The listing builds one solid part. Answer for the finished solid, in the listing's coordinates (mm). Face numbers are marked on the shaded views. A direction names the side the tool comes from. Give positions to 0.01 mm unless a question says otherwise; leave off trailing zeros. Loops run counter-clockwise (first coordinate to the right, second up) from the corner with the lowest first, then second, coordinate; pieces in that order, holes last. Notation, with made-up numbers: M 31.5,-9 L 46.5,-9 A7 ccw 46.5,-2 Z; hole C 80,26.25 d3. An arc over 180 degrees is marked long. One line per item, written item: value. Start each with the question number.
Q1. A cutting plane is placed at C-C, the plane y = 9. Determine the outline of the cut face in (x, z) (3 decimals), and give its area (3 significant figures).
Q2. A cutting plane is placed at D-D, the plane x = -21.5. Determine the outline of the cut face in (y, z).
Q3. The mould has two halves that part along Y. Classify the marked faces 1, 2 and 3: +Y half, -Y half, draft (parallel to the pull), parting line (faces both ways), or undercut.
Q4. Flat-ended cylindrical pins translate along their axes: pin 1 (2 mm diameter, centred on x = -3.5, y = 6.5, fed in from -Z); pin 2 (2 mm diameter, centred on x = 0, y = 6, fed in from +Z); pin 3 (4 mm diameter, centred on y = 8.5, z = -11, fed in from +X). Find the tip coordinate at first contact, or state that the pin passes through.
Q5. Consider L1, parallel to Y at x = -12, z = -20; L2, parallel to Z at x = -19, y = 9.5; L3, parallel to Z at x = 16.5, y = 6.75. Determine where each line is inside the solid, lowest interval first.
Q6. For the marked faces 4 and 5, determine the directions among +Z, -Z, +X, -X, +Y, -Y from which every point of the face is accessible in a straight line to the end or side of a thin tool.
Autodesk Fusion 360 part; units mm, degrees
sketch "Base" plane through (0, 0, 0) normal (0, 1, 0) x (1, 0, 0)
  circle A0 centre (0, 0) radius 25.4
  dimension "d1" = 50.8
extrude "Extrude1" add sketch "Base" along normal blind 12.7 makes body 1
sketch "Relief" plane through (0, 12.7, 0) normal (0, 1, 0) x (-1, 0, 0)
  circle A0 centre (0, 0) radius 25.4
  circle A1 centre (0, -25.4) radius 9.525
  dimension "d4" = 19.05
extrude "Extrude2" cut sketch "Relief" against normal blind 6.35 contours A0 A1 | A0 A1 picked at (1.7493, -22.2335) picked at (2.3346, -28.2419) bodies 1
sketch "Boss Ref" plane through (0, 12.7, 0) normal (0, 1, 0) x (-1, 0, 0)
  arc A0 (9.3561, -23.6141) -> (-9.3561, -23.6141) centre (0, -25.4) ccw
  arc A1 (9.3561, -23.6141) -> (-9.3561, -23.6141) centre (0, 0) ccw
  circle A2 centre (0, -10.795) radius 4.7625
  circle A3 centre (0, -10.795) radius 2.5527
  dimension "d7" = 9.525
  dimension "d8" = 10.795
  dimension "d9" = 5.1054
sketch "Revolve Cut1" plane through (0, 0, 0) normal (1, 0, 0) x (0, 0, -1)
  line L0 (25.4, 0) -> (25.4, 6.35)
  line L1 (-25.4, 12.7) -> (-25.4, 0)
  line L2 (15.875, 6.35) -> (23.6141, 6.35)
  line L3 (25.4, 6.35) -> (22.225, 6.35)
  line L4 (22.225, 7.9375) -> (25.4, 7.9375)
  line L5 (25.4, 7.9375) -> (25.4, 6.35)
  line L6 (22.225, 7.9375) -> (22.225, 6.35)
  dimension "d12" = 3.175
  dimension "d13" = 1.5875
revolve "Revolve1" cut sketch "Revolve Cut1" angle 360 about axis through (0, 1.75, 0) along (0, 1, 0) bodies 1
sketch "Sketch5" plane through (0, 12.7, 0) normal (0, 1, 0) x (-1, 0, 0)
  arc A0 (9.3561, -23.6141) -> (-9.3561, -23.6141) centre (0, -25.4) ccw
  arc A1 (9.3561, -23.6141) -> (-9.3561, -23.6141) centre (0, 0) ccw
  arc A2 (-8.2489, -20.6375) -> (-9.3561, -23.6141) centre (0, -25.4) ccw
  arc A3 (9.3561, -23.6141) -> (-9.3561, -23.6141) centre (0, 0) ccw
  arc A4 (9.3561, -23.6141) -> (8.2489, -20.6375) centre (0, -25.4) ccw
  arc A5 (8.2489, -20.6375) -> (-8.2489, -20.6375) centre (0, 0) ccw
  line L0 (0, -15.875) -> (-6.35, -9.525)
  line L1 (0, -15.875) -> (6.35, -9.525)
  line L2 (6.35, -9.525) -> (-6.35, -9.525)
  line L3 (0, -9.525) -> (0, -15.875) construction
  line L4 (6.35, -3.175) -> (-6.35, -3.175)
  line L5 (6.35, -9.525) -> (6.35, -3.175)
  line L6 (-6.35, -9.525) -> (-6.35, -3.175)
  line L7 (-6.35, -3.175) -> (-12.7, -3.175)
  line L8 (-12.7, -3.175) -> (-6.35, -9.525)
  line L9 (6.35, -9.525) -> (12.7, -3.175)
  line L10 (12.7, -3.175) -> (6.35, -3.175)
  dimension "d15" = 6.35
  dimension "d16" = 45
  dimension "d17" = 6.35
ref_plane "WorkPlane1" through (0, 0, -23.6141) normal (0, 0, 1) x (1, 0, 0)
sketch "Loft Profile 2" plane through (0, 12.7, 0) normal (0, 1, 0) x (-1, 0, 0)
  arc A0 (9.3561, -23.6141) -> (-9.3561, -23.6141) centre (0, -25.4) ccw
  arc A1 (9.3561, -23.6141) -> (-9.3561, -23.6141) centre (0, 0) ccw
  line L0 (4.7625, 8.255) -> (-4.7625, 8.255)
  arc A2 (-4.7625, 8.255) -> (-4.7625, -8.255) centre (-4.7625, 0) ccw
  line L1 (-4.7625, -8.255) -> (4.7625, -8.255)
  arc A3 (4.7625, -8.255) -> (4.7625, 8.255) centre (4.7625, 0) ccw
  line L2 (4.7625, 0) -> (-4.7625, 0) construction
  dimension "d19" = 9.525
  dimension "d20" = 8.255
sketch "Loft Profile 1" plane through (0, 0, 0) normal (0, -1, 0) x (1, 0, 0)
  circle A0 centre (0, 0) radius 25.4
  circle A1 centre (0, 0) radius 6.35
  dimension "d21" = 12.7
sketch "Sweep Profile" plane through (0, 0, 0) normal (0, -1, 0) x (1, 0, 0)
  circle A0 centre (0, 0) radius 25.4
  circle A1 centre (0, 0) radius 19.05
  dimension "d22" = 38.1
sketch "Sweep Path" plane through (0, 0, 0) normal (0, 0, 1) x (1, 0, 0)
  line L0 (0, 0) -> (0, -63.5)
  arc A0 (0, -63.5) -> (50.1381, -135.1046) centre (76.2, -63.5) ccw
  line L1 (50.1381, -135.1046) -> (169.479, -178.5411)
  dimension "d23" = 76.2
  dimension "d24" = 63.5
  dimension "d25" = 127
  dimension "d26" = 110
sketch "Hole Loc1" plane through (0, 12.7, 0) normal (0, 1, 0) x (-1, 0, 0)
  arc A0 (9.3561, -23.6141) -> (-9.3561, -23.6141) centre (0, -25.4) ccw
  arc A1 (9.3561, -23.6141) -> (-9.3561, -23.6141) centre (0, 0) ccw
  line L0 (0, 0) -> (0, -15.875) construction
  line L1 (0, 0) -> (-11.2253, -11.2253) construction
  point P0 (-11.2253, -11.2253)
  point P1 (11.2253, -11.2253)
  point P2 (11.2253, 11.2253)
  point P3 (-11.2253, 11.2253)
  dimension "d27" = 45
  dimension "d29" = 360
sketch "Extrude" plane through (0, 12.7, 0) normal (0, 1, 0) x (-1, 0, 0)
  arc A0 (9.3561, -23.6141) -> (-9.3561, -23.6141) centre (0, -25.4) ccw
  arc A1 (9.3561, -23.6141) -> (-9.3561, -23.6141) centre (0, 0) ccw
  line L0 (3.175, -16.4197) -> (-3.175, -16.4197)
  line L1 (-3.175, -16.4197) -> (-3.175, -9.525)
  line L2 (-3.175, -9.525) -> (3.175, -9.525)
  line L3 (3.175, -9.525) -> (3.175, -16.4197)
  line L4 (0, -9.525) -> (0, -15.875) construction
  dimension "d30" = 6.35
  dimension "d31" = 6.35
sketch "Revolve Cut2" plane through (0, 0, 0) normal (1, 0, 0) x (0, 0, -1)
  line L0 (25.4, 3.175) -> (22.225, 3.175)
  line L1 (22.225, 3.175) -> (22.225, 1.5875)
  line L2 (22.225, 1.5875) -> (25.4, 1.5875)
  line L3 (25.4, 1.5875) -> (25.4, 3.175)
  line L4 (25.4, 0) -> (25.4, 6.35)
  line L5 (22.225, 7.9375) -> (22.225, 6.35)
sketch "New Body" plane through (0, 12.7, 0) normal (0, 1, 0) x (-1, 0, 0)
  arc A0 (-4.7625, 8.255) -> (-4.7625, -8.255) centre (-4.7625, 0) ccw
  line L0 (-4.7625, -8.255) -> (4.7625, -8.255)
  arc A1 (4.7625, -8.255) -> (4.7625, 8.255) centre (4.7625, 0) ccw
  line L1 (4.7625, 8.255) -> (-4.7625, 8.255)
  line L2 (-4.7625, -9.525) -> (4.7625, -9.525)
  arc A2 (4.7625, -9.525) -> (4.7625, 9.525) centre (4.7625, 0) ccw
  line L3 (4.7625, 9.525) -> (-4.7625, 9.525)
  arc A3 (-4.7625, 9.525) -> (-4.7625, -9.525) centre (-4.7625, 0) ccw
  dimension "d32" = 1.27
extrude "Extrude4" add sketch "New Body" along normal blind 6.35 separate body contours A0 L0 A1 L1 | L2 A2 L3 A3 makes body 2
sketch "Sweep Guide" plane through (0, 0, 0) normal (0, 0, 1) x (1, 0, 0)
  line L0 (-25.4, 0) -> (25.4, 0)
  line L1 (25.4, 0) -> (25.4, -63.5)
  arc A0 (25.4, -63.5) -> (76.2, -114.3) centre (76.2, -63.5) ccw
  line L2 (76.2, -114.3) -> (169.479, -114.3)
  point P0 (76.2, -63.5)
  point P1 (169.479, -178.5411)
hidden bodies 2
equation "d17 = d15"
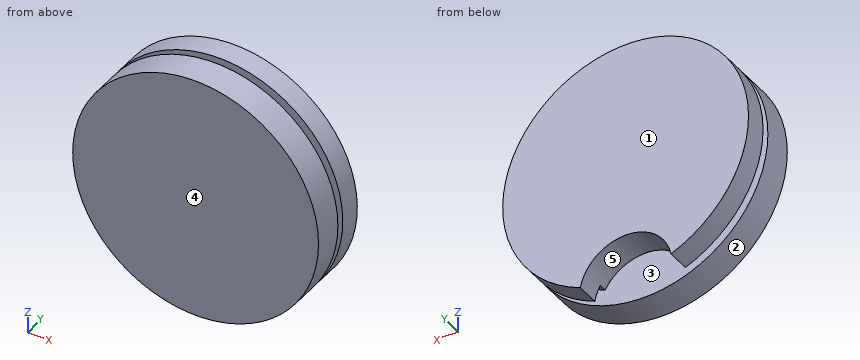
Answer block:
1. outline: M -9.356,-23.614 A9.525 cw 9.356,-23.614 A25.4 ccw long Z
1. area: 1,900 mm^2
2. outline: M 0,-13.52 L 6.35,-13.52 L 6.35,-5.63 L 7.94,-5.63 L 7.94,-13.52 L 12.7,-13.52 L 12.7,13.52 L 7.94,13.52 L 7.94,5.63 L 6.35,5.63 L 6.35,13.52 L 0,13.52 Z
3. face 1: +Y half
3. face 2: draft
3. face 3: undercut
4. pin 1: z = -25.28
4. pin 2: z = 25.4
4. pin 3: x = 23.75
5. L1: 0 to 6.35, 7.94 to 12.7
5. L2: -16.86 to 16.86
5. L3: -14.89 to 14.89
6. face 4: +Z, -Z, +X, -X, -Y
6. face 5: -Z, +Y
